from build123d import *

# Parameters (mm, degrees)
BOSS_EXTRUDE1_DEPTH = 15
SKETCH2_W           = 10
SKETCH2_H           = 5
CUT_EXTRUDE1_DEPTH  = 5
SKETCH3_W           = 5
SKETCH3_H           = 5
CUT_EXTRUDE2_DEPTH  = 10


with BuildPart() as part:
    # Sketch1 → Boss-Extrude1 (new body)
    with BuildSketch(Plane.XY):
        Polygon((0, 0), (0, 15), (-5, 15), (-5, 10), (-10, 10), (-10, 5), (-15, 5), (-15, 0), align=None)
    extrude(amount=BOSS_EXTRUDE1_DEPTH)

    # Sketch2 → Cut-Extrude1 (cut)
    with BuildSketch(Plane.XY.offset(15)):
        with Locations((-5, 7.5)):
            Rectangle(SKETCH2_W, SKETCH2_H)
    extrude(amount=-CUT_EXTRUDE1_DEPTH, mode=Mode.SUBTRACT)

    # Sketch3 → Cut-Extrude2 (cut)
    with BuildSketch(Plane.XY.offset(15)):
        with Locations((-2.5, 12.5)):
            Rectangle(SKETCH3_W, SKETCH3_H)
    extrude(amount=-CUT_EXTRUDE2_DEPTH, mode=Mode.SUBTRACT)


solid = part.part
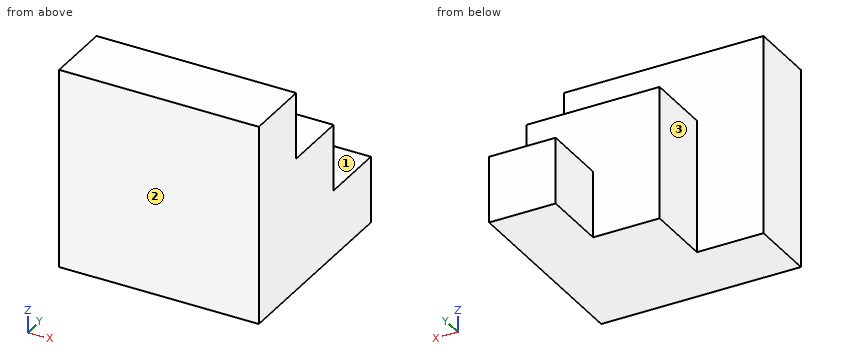
Input: part model. Units: mm. Frame: model coordinates. Face numbers are marked on the shaded views. A direction names the side the tool comes from. Coordinates: 2 decimals unless noted, no trailing zeros. Loops run counter-clockwise (first coordinate to the right, second up) from the corner with the lowest first, then second, coordinate; pieces in that order, holes last. Notation, with made-up numbers: (-21, 54) - (19, 54) arc R5 ccw to (19, 60) - close; hole circle Ø11 at (81.5, -4.5). An arc over 180 degrees is marked (long way). Answer in a Markdown table with one row per item. Add a question column.
Item 1: Section query C-C on y = 13.75. Return the cut outline in (x, z).
Item 2: Line query: line 1 along Z through (x, y) = (-3.75, 14); line 2 along X through (y, z) = (8.5, 5). Output: solid intervals per line, ascending. Write a range as [from, to].
Item 3: Section query A-A on x = -6. Return the cut outline in (y, z), then the cut area to 3 significant figures.
Item 4: Access query for the marked faces 1, 2 and 3. Directions: +Z, -Z, +X, -X, +Y, -Y. A direction counts if a zero-diameter tool reaches every point of the face in a straight line with its end or side. Return the directions, or none.
Item 5: Section query B-B on z = 13. Return the cut outline in (x, y).
Item 6: Section query D-D on x = -3.5. Return the cut outline in (y, z), then the cut area to 3 significant figures.
Item 7: Contact query for flat-ended pins moving along their axis: P1, Ø6, axis at y = 9, z = 3, coming from the +X side; P2, Ø6, axis at x = -5, z = 9, coming from the +Y side; P3, Ø5.5, axis at y = 13.5, z = 1.5, coming from the -X side; P4, Ø2.5, axis at y = 7, z = 7, coming from the -X side. Output: stop coordinate, or through.
Recorded:
| question | item | result |
|---|---|---|
| 1 | outline | (-5, 0) - (0, 0) - (0, 5) - (-5, 5) - close |
| 2 | line 1 | [0, 5] |
| 2 | line 2 | [-10, 0] |
| 3 | outline | (0, 0) - (10, 0) - (10, 10) - (5, 10) - (5, 15) - (0, 15) - close |
| 3 | area | 125 mm^2 |
| 4 | face 1 | +Z, +X, -X, +Y |
| 4 | face 2 | +Z, -Z, +X, -X, -Y |
| 4 | face 3 | +Z, -Z, -X, +Y |
| 5 | outline | (-15, 0) - (0, 0) - (0, 5) - (-15, 5) - close |
| 6 | outline | (0, 0) - (15, 0) - (15, 5) - (10, 5) - (10, 10) - (5, 10) - (5, 15) - (0, 15) - close |
| 6 | area | 150 mm^2 |
| 7 | P1 | x = 0 |
| 7 | P2 | y = 10 |
| 7 | P3 | x = -5 |
| 7 | P4 | x = -10 |
